Autodesk Inventor part; units mm, degrees
ref_plane "YZ Plane" through (0, 0, 0) normal (1, 0, 0) x (0, 1, 0)
ref_plane "XZ Plane" through (0, 0, 0) normal (0, 1, 0) x (-1, 0, 0)
ref_plane "XY Plane" through (0, 0, 0) normal (0, 0, 1) x (1, 0, 0)
sketch "Sketch1" plane through (0, 0, 0) normal (0, 0, 1) x (1, 0, 0)
  line L0 (9.398, 0) -> (41.402, 0)
  line L1 (50.8, 9.398) -> (50.8, 50.8)
  line L2 (50.8, 50.8) -> (46.228, 50.8)
  line L3 (46.228, 50.8) -> (46.228, 9.398)
  line L4 (41.402, 4.572) -> (9.398, 4.572)
  line L5 (4.572, 9.398) -> (4.572, 50.8)
  line L6 (4.572, 50.8) -> (0, 50.8)
  line L7 (0, 50.8) -> (0, 9.398)
  arc A0 (4.572, 9.398) -> (9.398, 4.572) centre (9.398, 9.398) ccw
  arc A1 (41.402, 4.572) -> (46.228, 9.398) centre (41.402, 9.398) ccw
  arc A2 (0, 9.398) -> (9.398, 0) centre (9.398, 9.398) ccw
  arc A3 (41.402, 0) -> (50.8, 9.398) centre (41.402, 9.398) ccw
  point P0 (0, 0)
  point P1 (50.8, 0)
  dimension "d0" = 50.8
  dimension "d1" = 50.8
  dimension "d2" = 4.572
  dimension "d3" = 4.572
  dimension "d4" = 4.572
  dimension "d5" = 4.826
  dimension "d6" = 9.398
extrude "Extrusion1" add sketch "Sketch1" against normal blind 76.2
fillet "Fillet1" radius 6.35 4 edges at (2.286, 50.8, 0) (48.514, 50.8, 0) (2.286, 50.8, -76.2) (48.514, 50.8, -76.2)
sketch "Sketch2" plane through (50.8, 9.398, 0) normal (1, 0, 0) x (0, 0, -1)
  line L0 (6.35, 41.402) -> (69.85, 41.402)
  line L1 (0, -9.398) -> (76.2, -9.398)
  point P0 (38.1, 22.352)
  point P1 (38.1, 41.402)
  dimension "d10" = 31.75
hole "Hole1" at (50.8, 31.75, -38.1) direction (-1, 0, 0) diameter 6.858 end through all
ref_plane "Work Plane1" through (25.4, 9.398, 0) normal (1, 0, 0) x (0, 0, -1)
ref_plane "Work Plane2" through (0, 0, -38.1) normal (0, 0, -1) x (-1, 0, 0)
equation "\"d3\" = d2"
equation "\"d4\" = d2"
properties part number "GE-13025-02" material "Steel"
Geometry check sheet. Reference: the model listing, model coordinates, mm. A direction names the side the tool comes from. Give positions to 0.01 mm unless a question says otherwise; leave off trailing zeros. Loops run counter-clockwise (first coordinate to the right, second up) from the corner with the lowest first, then second, coordinate; pieces in that order, holes last. Notation, with made-up numbers: M 11,79 L 21,79 A20 ccw 21,85 Z; hole C 1.25,32 d6. An arc over 180 degrees is marked long. Answer as CSV lines item,"result".
Item 1: Cross-section at B-B on z = -38.1. Record the cut outline in (x, y), and give its area (3 significant figures).
Values:
outline,"M 0,9.4 A9.4 ccw 9.4,0 L 41.4,0 A9.4 ccw 50.8,9.4 L 50.8,28.32 L 46.23,28.32 L 46.23,9.4 A4.83 cw 41.4,4.57 L 9.4,4.57 A4.83 cw 4.57,9.4 L 4.57,28.32 L 0,28.32 Z; M 0,35.18 L 4.57,35.18 L 4.57,50.8 L 0,50.8 Z; M 46.23,35.18 L 50.8,35.18 L 50.8,50.8 L 46.23,50.8 Z"
area,"564 mm²"
Item 2: Depth check by flat-ended pin: P1, Ø1, axis at x = 17.5, z = -20, coming from the +Y side; P2, Ø5, axis at x = 35.5, y = 9.5, coming from the +Z side. Enter the tip coordinate at first touch or a pass-through.
Values:
P1,"stops at y = 4.57"
P2,"passes through"
Item 3: Cross-section at D-D on z = -22.5. Record the cut outline in (x, y), and give its area (3 significant figures).
Values:
outline,"M 0,9.4 A9.4 ccw 9.4,0 L 41.4,0 A9.4 ccw 50.8,9.4 L 50.8,50.8 L 46.23,50.8 L 46.23,9.4 A4.83 cw 41.4,4.57 L 9.4,4.57 A4.83 cw 4.57,9.4 L 4.57,50.8 L 0,50.8 Z"
area,"627 mm²"
Item 4: Release check for a two-part mould opening along X. For faces 3 (the flat face through (0, 26, -38)), 4 (the flat face through (25, 0, -38)), 5 (the flat face through (50.8, 25, -38)), 6 (the flat face through (46.228, 26, -38)) record: pulls with the +X half, pulls with the -X half, needs draft (parallel to the pull), parting line crosses it, or undercut.
Values:
face 3,"pulls with the -X half"
face 4,"needs draft"
face 5,"pulls with the +X half"
face 6,"undercut"
Item 5: Cross-section at C-C on y = 48.5. Record the cut outline in (x, z).
Values:
outline,"M 0,-74.74 L 4.57,-74.74 L 4.57,-1.46 L 0,-1.46 Z; M 46.23,-74.74 L 50.8,-74.74 L 50.8,-1.46 L 46.23,-1.46 Z"
Item 6: Access from +Z, -Z, +X, -X, +Y, -Y to the whole of each face (thin tool, end or side, straight path). Record for faces 1 (the flat face through (26, 4.572, -38)), 2 (the cylindrical face through (2.25, 48.99, -74.29)).
Values:
face 1,"+Z, -Z, +Y"
face 2,"-Z, +X, -X, +Y"
Item 7: Material ranges on line 1 (X direction, y = 31, z = -5); line 2 (Y direction, x = 21.5, z = -33.5); line 3 (Z direction, x = 1.55, y = 31.75), recorded low to high.
Values:
line 1,"x = 0 to 4.57, 46.23 to 50.8"
line 2,"y = 0 to 4.57"
line 3,"z = -76.2 to -41.53, -34.67 to 0"
Item 8: Cross-section at A-A on y = 31.75. Record the cut outline in (x, z), and give its area (3 significant figures).
Values:
outline,"M 0,-76.2 L 4.57,-76.2 L 4.57,-41.53 L 0,-41.53 Z; M 0,-34.67 L 4.57,-34.67 L 4.57,0 L 0,0 Z; M 46.23,-76.2 L 50.8,-76.2 L 50.8,-41.53 L 46.23,-41.53 Z; M 46.23,-34.67 L 50.8,-34.67 L 50.8,0 L 46.23,0 Z"
area,"634 mm²"
